Here's how the part is built. I have some questions about the finished solid (model axes, mm). Face numbers are marked on the shaded views. A direction names the side the tool comes from. Coordinates: 2 decimals unless noted, no trailing zeros. Order: outer loops, then holes, each group sorted by start corner. A loop starts at its lowest first (then second) coordinate and runs counter-clockwise, first axis right, second up. Notation, with made-up numbers: (71.5, 46.25) - (93.5, 46.25) arc R17 cw to (93.5, 59.25) - close; hole circle Ø1 at (79, 50.25). An arc over 180 degrees is marked (long way). Use CSV: the item, a comma, the result in double quotes. Start each with the question number.
from build123d import *

# Parameters (mm, degrees)
F0_W     = 127
F0_H     = 114.6371724766
F1_DEPTH = 103.124
F3_D     = 25.4
F4_R     = 6.35
F5_T     = -2.54


with BuildPart() as f1:
    # F0 (on Top) → F1 (new body)
    with BuildSketch(Plane.XY):
        with Locations((-0.032884495, 0.0296833506)):
            Rectangle(F0_W, F0_H)
    extrude(amount=F1_DEPTH)

    # F3 (through all)
    with Locations(Plane.XY.offset(103.124)):
        with Locations((0, 0)):
            Hole(F3_D / 2)

    # F4
    f4_edges = [f1.edges().sort_by_distance(p)[0] for p in [
        (-0.032884, 57.34827, 103.124),
        (63.467116, 0.029683, 103.124),
        (-63.532884, 0.029683, 103.124),
        (-0.032884, -57.288903, 103.124),
        (-12.7, 0, 103.124),
    ]]
    fillet(f4_edges, radius=F4_R)

    # F5
    f5_openings = [f1.faces().sort_by_distance(p)[0] for p in [
        (-0.032884, 55.637402, 0),
    ]]
    offset(amount=F5_T, openings=f5_openings)


solid = f1.part
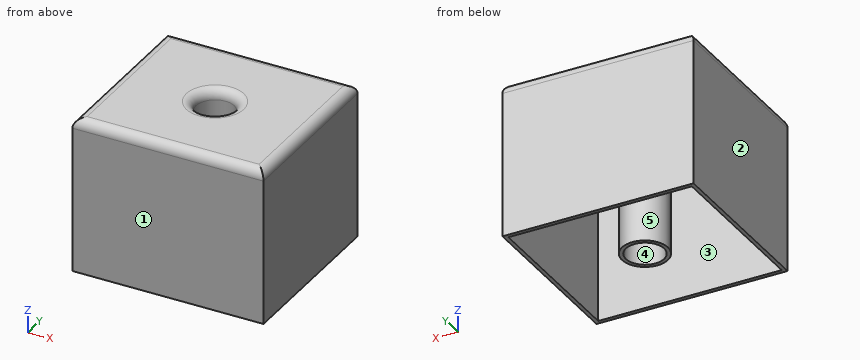
Item 1: For pin 1 Ø2 at (x, y) = (6.5, 7.5) entering from -Z; pin 2 Ø3 at (x, y) = (16, 43.5) entering from -Z, each with a flat end and sliding along its axis, tell me the tip position at first contact or that it passes through.
Item 2: Please list where these lines run through material, in increasing order: line 1 along Y through (x, z) = (0, 37); line 2 along X through (y, z) = (-47, 34); line 3 along Y through (x, z) = (-13, 21). Write a range as from..to.
Item 3: We'd pull the mould along X, two halves only. Please class the marked faces 1, 2 and 3: released by +X, released by -X, zero draft, split by the parting line, or undercut.
Item 4: Suppose I cut it at D-D on x = -31. Write out the boundary of the cut face in (y, z).
Item 5: Suppose I cut it at A-A on z = 67.5. Write out the boundary of the cut face in (x, y).
Item 6: Suppose I cut it at C-C on y = 0. Write out the boundary of the cut face in (x, z), then the cut area to 3 significant figures.
Item 7: Suppose I cut it at B-B on x = 0. Write out the boundary of the cut face in (y, z).
Item 8: For the marked faces 4 and 5, which set-ups out of +Z, -Z, +X, -X, +Y, -Y let a thin tool reach every point of the face, with its end or its side?
Here are the results:
1,pin 1,"through"
1,pin 2,"z = 100.58"
2,line 1,"-57.29..-54.75, -15.24..-12.7, 12.7..15.24, 54.81..57.35"
2,line 2,"-63.53..-60.99, 60.93..63.47"
2,line 3,"-57.29..-54.75, -7.95..7.95, 54.81..57.35"
3,face 1,"zero draft"
3,face 2,"released by -X"
3,face 3,"undercut"
4,outline,"(-57.29, 0) - (-54.75, 0) - (-54.75, 96.77) arc R3.81 cw to (-50.94, 100.58) - (51, 100.58) arc R3.81 cw to (54.81, 96.77) - (54.81, 0) - (57.35, 0) - (57.35, 96.77) arc R6.35 ccw to (51, 103.12) - (-50.94, 103.12) arc R6.35 ccw to (-57.29, 96.77) - close"
5,outline,"(-63.53, -57.29) - (63.47, -57.29) - (63.47, 57.35) - (-63.53, 57.35) - close; circle Ø30.48 at (0, 0); hole (-60.99, -54.75) - (60.93, -54.75) - (60.93, 54.81) - (-60.99, 54.81) - close; hole circle Ø25.4 at (0, 0)"
6,outline,"(-63.53, 0) - (-60.99, 0) - (-60.99, 96.77) arc R3.81 cw to (-57.18, 100.58) - (-19.05, 100.58) arc R3.81 cw to (-15.24, 96.77) - (-15.24, 0) - (-12.7, 0) - (-12.7, 96.77) arc R6.35 ccw to (-19.05, 103.12) - (-57.18, 103.12) arc R6.35 ccw to (-63.53, 96.77) - close; (12.7, 0) - (15.24, 0) - (15.24, 96.77) arc R3.81 cw to (19.05, 100.58) - (57.12, 100.58) arc R3.81 cw to (60.93, 96.77) - (60.93, 0) - (63.47, 0) - (63.47, 96.77) arc R6.35 ccw to (57.12, 103.12) - (19.05, 103.12) arc R6.35 ccw to (12.7, 96.77) - close"
6,area,"1,260 mm^2"
7,outline,"(-57.29, 0) - (-54.75, 0) - (-54.75, 96.77) arc R3.81 cw to (-50.94, 100.58) - (-19.05, 100.58) arc R3.81 cw to (-15.24, 96.77) - (-15.24, 0) - (-12.7, 0) - (-12.7, 96.77) arc R6.35 ccw to (-19.05, 103.12) - (-50.94, 103.12) arc R6.35 ccw to (-57.29, 96.77) - close; (12.7, 0) - (15.24, 0) - (15.24, 96.77) arc R3.81 cw to (19.05, 100.58) - (51, 100.58) arc R3.81 cw to (54.81, 96.77) - (54.81, 0) - (57.35, 0) - (57.35, 96.77) arc R6.35 ccw to (51, 103.12) - (19.05, 103.12) arc R6.35 ccw to (12.7, 96.77) - close"
8,face 4,"+Z, -Z"
8,face 5,"-Z"
